Check sheet for the drawn part. Datum: minimum x, y, z corner. Units: mm. Coordinates: 2 decimals unless noted, no trailing zeros. Write each loop counter-clockwise with the first axis right and the second up, starting at its lowest first coordinate (ties: lowest second). Pieces come first, ordered by that corner, then holes. Notation, with made-up numbers: (29.5, -14) -> (66.5, -14) arc R12 ccw to (66.5, 6) -> close; hole circle Ø9 at (-33, 2.5). An arc over 180 degrees is marked (long way). Answer in a Markdown table with one row per item.
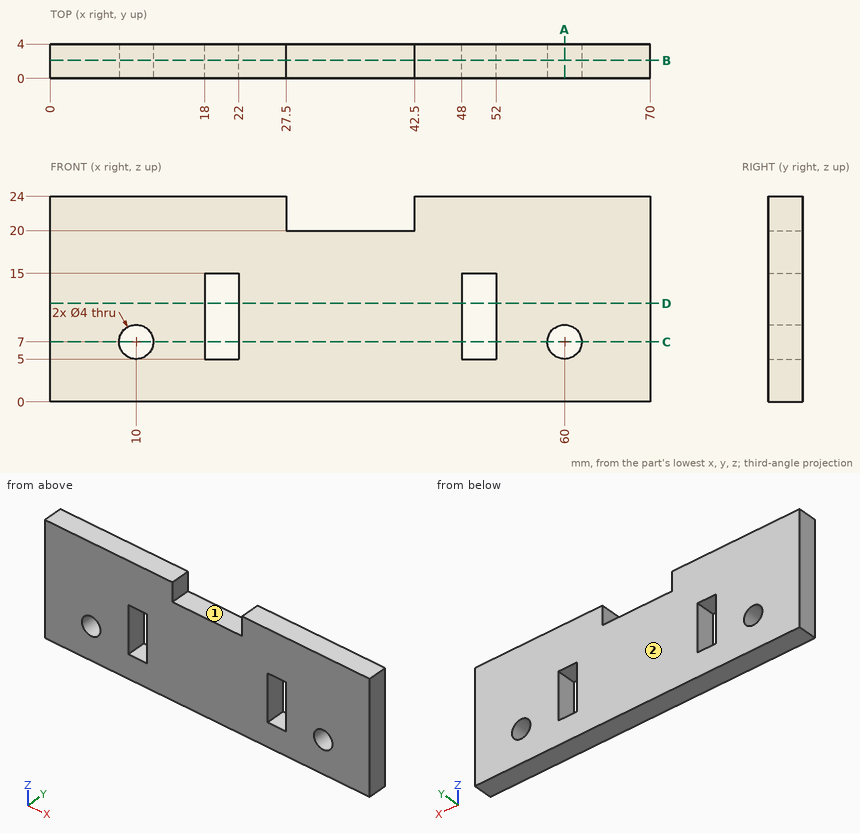
1. Sectioned sample at B-B, the plane y = 2.1. Record the cut outline in (x, z).
Findings below:
| item | result |
|---|---|
| outline | (0, 0) -> (70, 0) -> (70, 24) -> (42.5, 24) -> (42.5, 20) -> (27.5, 20) -> (27.5, 24) -> (0, 24) -> close; hole circle Ø4 at (10, 7); hole (18, 5) -> (22, 5) -> (22, 15) -> (18, 15) -> close; hole (48, 5) -> (52, 5) -> (52, 15) -> (48, 15) -> close; hole circle Ø4 at (60, 7) |
2. Sectioned sample at A-A, the plane x = 60. Record the cut outline in (y, z).
Findings below:
| item | result |
|---|---|
| outline | (0, 0) -> (4, 0) -> (4, 5) -> (0, 5) -> close; (0, 9) -> (4, 9) -> (4, 24) -> (0, 24) -> close |
3. Material ranges on probe 1 along X at (y, z) = (0.7, 10.5); probe 2 along X at (y, z) = (2, 7); probe 3 along Z at (x, y) = (60, 2), recorded low to high. Write a range as from..to.
Findings below:
| item | result |
|---|---|
| probe 1 | x = 0..18, 22..48, 52..70 |
| probe 2 | x = 0..8, 12..18, 22..48, 52..58, 62..70 |
| probe 3 | z = 0..5, 9..24 |
4. Sectioned sample at D-D, the plane z = 11.5. Record the cut outline in (x, y).
Findings below:
| item | result |
|---|---|
| outline | (0, 0) -> (18, 0) -> (18, 4) -> (0, 4) -> close; (22, 0) -> (48, 0) -> (48, 4) -> (22, 4) -> close; (52, 0) -> (70, 0) -> (70, 4) -> (52, 4) -> close |
5. Sectioned sample at C-C, the plane z = 7. Record the cut outline in (x, y), and give its area (3 significant figures).
Findings below:
| item | result |
|---|---|
| outline | (0, 0) -> (8, 0) -> (8, 4) -> (0, 4) -> close; (12, 0) -> (18, 0) -> (18, 4) -> (12, 4) -> close; (22, 0) -> (48, 0) -> (48, 4) -> (22, 4) -> close; (52, 0) -> (58, 0) -> (58, 4) -> (52, 4) -> close; (62, 0) -> (70, 0) -> (70, 4) -> (62, 4) -> close |
| area | 216 mm² |
6. Release check for a two-part mould opening along X. For the marked faces 1 and 2 record: released by +X, released by -X, zero draft, split by the parting line, or undercut.
Findings below:
| item | result |
|---|---|
| face 1 | undercut |
| face 2 | zero draft |
7. Go/stop test with a flat-tipped pin: pin 1 (2 mm diameter, centred on x = 38, y = 2, fed in from +Z). Record where the tip stops, or that it passes through.
Findings below:
| item | result |
|---|---|
| pin 1 | stops at z = 20 |
